from build123d import *

# Parameters (mm, degrees)
EXTRUDE_1_DEPTH = 56.773811


with BuildPart() as part:
    # Эскиз1 → Бобышка-Вытянуть1 (new body)
    with BuildSketch(Plane(origin=(0, 0, 0), x_dir=(1, 0, 0), z_dir=(0, 1, 0))):
        with BuildLine():
            Line((-27, 15), (-3, 15))
            ThreePointArc((-3, 15), (-0.878679656, 14.121320344), (0, 12))
            Line((0, 12), (0, -12))
            ThreePointArc((0, -12), (-0.878679656, -14.121320344), (-3, -15))
            Line((-3, -15), (-27, -15))
            ThreePointArc((-27, -15), (-29.121320344, -14.121320344), (-30, -12))
            Line((-30, -12), (-30, 12))
            ThreePointArc((-30, 12), (-29.121320344, 14.121320344), (-27, 15))
        make_face()
        with BuildLine():
            Line((-26, 13), (-4, 13))
            ThreePointArc((-4, 13), (-2.585786438, 12.414213562), (-2, 11))
            Line((-2, 11), (-2, -11))
            ThreePointArc((-2, -11), (-2.585786438, -12.414213562), (-4, -13))
            Line((-4, -13), (-26, -13))
            ThreePointArc((-26, -13), (-27.414213562, -12.414213562), (-28, -11))
            Line((-28, -11), (-28, 11))
            ThreePointArc((-28, 11), (-27.414213562, 12.414213562), (-26, 13))
        make_face(mode=Mode.SUBTRACT)
    extrude(amount=-EXTRUDE_1_DEPTH)


solid = part.part
Geometry: final body of the model. Coordinates: model frame, mm. A direction names the side the tool comes from. Give positions to 0.01 mm unless a question says otherwise; leave off trailing zeros. Loops run counter-clockwise (first coordinate to the right, second up) from the corner with the lowest first, then second, coordinate; pieces in that order, holes last. Notation, with made-up numbers: M -36,54.25 L -23,54.25 A27 ccw -23,70.25 Z; hole C 49,73 d2. An arc over 180 degrees is marked long. Put each result on its own line as item: value. Start each with the question number.
1) Pull-direction query (Z, two-part tool) for faces 3 (the flat face through (-1, -56.774, 0)), 4 (the flat face through (-15, -28, -13)), 5 (the flat face through (-15, -28, 15)); classes: pulls with the +Z half, pulls with the -Z half, needs draft (parallel to the pull), parting line crosses it, or undercut.
2) Ray query, line 1 along X through (y, z) = (-10.5, 4); line 2 along Z through (x, y) = (-13, -14); line 3 along X through (y, z) = (-41, 12.5). Return the intervals inside material, ascending.
3) Cut plane A-A (z = 7). Output: boundary loops of the cut face in (x, y), then the cut area to 3 significant figures.
4) Cut plane C-C (x = -17.5). Output: boundary loops of the cut face in (y, z), then the cut area to 3 significant figures.
5) Access query for faces 1 (the cylindrical face through (-27.43, -27.99, -12.4)), 2 (the flat face through (-1, 0, 0)). Directions: +Z, -Z, +X, -X, +Y, -Y. A direction counts if a zero-diameter tool reaches every point of the face in a straight line with its end or side. Return the directions, or none.
6) Cut plane B-B (y = -52). Output: boundary loops of the cut face in (x, z), then the cut area to 3 significant figures.
Verdict:
1. face 3: needs draft
1. face 4: undercut
1. face 5: pulls with the +Z half
2. line 1: -30 to -28, -2 to 0
2. line 2: -15 to -13, 13 to 15
2. line 3: -29.96 to -27.32, -2.68 to -0.04
3. outline: M -30,-56.77 L -28,-56.77 L -28,0 L -30,0 Z; M -2,-56.77 L 0,-56.77 L 0,0 L -2,0 Z
3. area: 227 mm2
4. outline: M -56.77,-15 L 0,-15 L 0,-13 L -56.77,-13 Z; M -56.77,13 L 0,13 L 0,15 L -56.77,15 Z
4. area: 227 mm2
5. face 1: +Y, -Y
5. face 2: +Z, -Z, +X, -X, +Y
6. outline: M -30,-12 A3 ccw -27,-15 L -3,-15 A3 ccw 0,-12 L 0,12 A3 ccw -3,15 L -27,15 A3 ccw -30,12 Z; hole M -28,-11 A2 ccw -26,-13 L -4,-13 A2 ccw -2,-11 L -2,11 A2 ccw -4,13 L -26,13 A2 ccw -28,11 Z
6. area: 220 mm2
